Autodesk Inventor part; units mm, degrees
ref_plane "YZ Plane" through (0, 0, 0) normal (1, 0, 0) x (0, 1, 0)
ref_plane "XZ Plane" through (0, 0, 0) normal (0, 1, 0) x (-1, 0, 0)
ref_plane "XY Plane" through (0, 0, 0) normal (0, 0, 1) x (1, 0, 0)
sketch "Skizze1" plane through (0, 0, 0) normal (0, 0, 1) x (1, 0, 0)
  line L0 (-523.9247, 0) -> (524.0578, 0)
  line L1 (0, -301.1361) -> (0, 1806.8169)
  line L2 (350, 0) -> (-350, 0) construction
  line L3 (-350, 0) -> (-374.2129, 6.2512)
  line L4 (-374.2129, 6.2512) -> (-24.346, 1505.6807)
  line L5 (-24.346, 1505.6807) -> (0, 1500)
  line L6 (350, 0) -> (374.346, 5.6807)
  line L7 (374.346, 5.6807) -> (24.346, 1505.6807)
  line L8 (24.346, 1505.6807) -> (0, 1500)
  line L9 (280, 300) -> (-280, 300)
  line L10 (274.1667, 325) -> (-274.1667, 325)
  line L11 (350, 0) -> (280, 300)
  line L12 (274.1667, 325) -> (0, 1500)
  line L13 (-350, 0) -> (-280, 300)
  line L14 (-274.1667, 325) -> (0, 1500)
  point P0 (0, 0)
  point P1 (0, 300)
  dimension "d9" = 700
  dimension "d11" = 300
  dimension "d18" = 1500
  dimension "d19" = 25
extrude "Extrusion2" add sketch "Skizze1" along normal blind 25 contours L3 L4 L5 L14 L10 L1 L9 L13 | L11 L9 L1 L10 L12 L8 L7 L6 | L10 L14 L1 | L1 L12 L10
extrude "Extrusion3" cut sketch "Skizze1" along normal through all contours L10 L14 L1 | L1 L12 L10
sketch "Skizze2" plane through (0, 0, 25) normal (0, 0, 1) x (1, 0, 0)
  circle A0 centre (0, 1520) radius 27.5
  circle A1 centre (0, 1520) radius 5.5
  line L0 (-274.1667, 325) -> (0, 1500)
  line L1 (0, 1500) -> (274.1667, 325)
  point P0 (0, 0)
  dimension "d38" = 55
  dimension "d39" = 1520
  dimension "d40" = 11
extrude "Extrusion4" add sketch "Skizze2" against normal blind 25
sketch "Skizze3" plane through (0, 0, 0) normal (0, 0, -1) x (-1, 0, 0)
  line L0 (24.346, 1505.6807) -> (374.2129, 6.2512)
  line L1 (350, 0) -> (280, 300)
  line L2 (374.2129, 6.2512) -> (350, 0)
  line L3 (332.9578, 73.0381) -> (357.3038, 78.7188)
  point P0 (0, 0)
  dimension "d44" = 75
extrude "Extrusion5" cut sketch "Skizze3" against normal blind 25
properties part number "Steher"
Could you check a few things on this model? Use its own coordinates, in mm. A direction names the side the tool comes from. Give positions to 0.01 mm unless a question says otherwise; leave off trailing zeros. Loops run counter-clockwise (first coordinate to the right, second up) from the corner with the lowest first, then second, coordinate; pieces in that order, holes last. Notation, with made-up numbers: (13, -29.75) -> (71, -29.75) arc R32 ccw to (71, 9.25) -> close; hole circle Ø2 at (-7.5, 86). An arc over 180 degrees is marked (long way). Return JSON: item names as keys, results as strings.
Item 1: We'd pull the mould along Y, two halves only. Please class faces 4 (the cylindrical face through (0.819, 1547.488, 12.675)), 5 (the flat face through (197, 663, 25)), 6 (the flat face through (-306.85, 184.93, 12.32)): +Y half, -Y half, draft (parallel to the pull), parting line (faces both ways), or undercut.
Geometry results:
{"face 4": "undercut", "face 5": "draft", "face 6": "-Y half"}
Item 2: Which directions (+Z, -Z, +X, -X, +Y, -Y) give clear straight access to the entire face, cutting with the end or side of a thin tool? Please do faces 1 (the flat face through (197, 663, 0)), 2 (the flat face through (315.49, 147.9, 12.32)), 3 (the flat face through (-139.86, 900.6, 12.32)).
Geometry results:
{"face 1": "-Z, +X, -X, +Y, -Y", "face 2": "+Z, -Z, -Y", "face 3": "+Z, -Z"}
Item 3: I'm going to push flat-ended pins straight in: pin 1 (1 mm diameter, centred on x = 203.5, z = 20, fed in from -Y); pin 2 (8 mm diameter, centred on y = 509, z = 13.5, fed in from +X); pin 3 (5 mm diameter, centred on y = 895.5, z = 2.5, fed in from +X). Where does each tip first touch, or does it pass through?
Geometry results:
{"pin 1": "stops at y = 300", "pin 2": "stops at x = 257.84", "pin 3": "stops at x = 167.3"}
Item 4: If we section it at B-B on z = 21: List the corners of the cut face in (x, y) for me.
Geometry results:
{"outline": "(-357.3, 78.72) -> (-332.96, 73.04) -> (-280, 300) -> (280, 300) -> (350, 0) -> (374.35, 5.68) -> (24.35, 1505.68) -> (23.33, 1505.44) arc R27.5 ccw (long way) to (-23.33, 1505.44) -> (-24.35, 1505.68) -> close; hole (-274.17, 325) -> (274.17, 325) -> (1.74, 1492.55) arc R27.5 cw to (-1.74, 1492.55) -> close; hole circle Ø11 at (0, 1520)"}
Item 5: If we section it at A-A on y = 1281: List the corners of the cut face in (x, z) for me.
Geometry results:
{"outline": "(-76.77, 0) -> (-51.1, 0) -> (-51.1, 25) -> (-76.77, 25) -> close; (51.1, 0) -> (76.77, 0) -> (76.77, 25) -> (51.1, 25) -> close"}
Item 6: If we section it at C-C on x = 129.5: List the corners of the cut face in (y, z) for me.
Geometry results:
{"outline": "(300, 0) -> (325, 0) -> (325, 25) -> (300, 25) -> close; (945, 0) -> (1055.02, 0) -> (1055.02, 25) -> (945, 25) -> close"}
Item 7: If we section it at D-D on x = 329: List the corners of the cut face in (y, z) for me, plus the area to 3 significant figures.
Geometry results:
{"outline": "(90, 0) -> (200.02, 0) -> (200.02, 25) -> (90, 25) -> close", "area": "2,750 mm²"}
Item 8: I need wall thicknesses on L1, parallel to Y at x = 0, z = 5.5; L2, parallel to X at y = 1520, z = 9.25; L3, parallel to X at y = 589, z = 6.25. Which ranges of each line are inside material? Lowest first, please. Write a range as from..to.
Geometry results:
{"L1": "y = 300..325, 1492.5..1514.5, 1525.5..1547.5", "L2": "x = -27.5..-5.5, 5.5..27.5", "L3": "x = -238.24..-212.57, 212.57..238.24"}
